Part model, mm, in its own coordinate system. Round coordinates to 2 decimals unless told otherwise and drop trailing zeros. Write each loop counter-clockwise with the first axis right and the second up, starting at its lowest first coordinate (ties: lowest second). Pieces come first, ordered by that corner, then holes. Notation, with made-up numbers: (-36.75, 35) -> (-30.75, 35) arc R16 cw to (-30.75, 50) -> close; hole circle Ø11 at (43.25, 78). An arc over 180 degrees is marked (long way). Return JSON: item names as keys, results as strings. Group by question number.
(1) Drop flat-ended pins along their axis: pin 1 Ø1 at (y, z) = (4, 23.5) entering from +X; pin 2 Ø2 at (y, z) = (2.5, -29) entering from -X; pin 3 Ø3 at (x, y) = (33.5, 4.5) entering from +Z; pin 4 Ø10 at (x, z) = (0, 31.75) entering from -Y. Give the stop position or say it passes through.
(2) Drill centre lines: L1, parallel to Z at x = 0.5, y = 4; L2, parallel to X at y = 2, z = 18.5; L3, parallel to Z at x = 4.5, y = 2.5. Where is each one in solid material? Low to high. Write a range as from..to.
(3) Saw through at A-A (z = 6.35). List the corners of the cut face in (x, y) (3 decimals).
from build123d import *

# Parameters (mm, degrees)
SKETCH1_R           = 3.175
SKETCH1_R_2         = 8.73125
BOSS_EXTRUDE1_DEPTH = 6.35
FILLET2_R           = 12.7
FILLET3_R           = 2.116666667
SKETCH2_R           = 10.2489
CUT_EXTRUDE1_DEPTH  = 1.27


with BuildPart() as part:
    # Sketch1 → Boss-Extrude1 (new body)
    with BuildSketch(Plane(origin=(0, 0, 0), x_dir=(1, 0, 0), z_dir=(0, 1, 0))):
        with BuildLine():
            Line((-12.7, 17.550968343), (-12.7, -44.45))
            Line((-12.7, -44.45), (12.7, -44.45))
            Line((12.7, -44.45), (12.7, 17.550968343))
            ThreePointArc((12.7, 17.550968343), (17.599905094, 24.459880613), (19.020487692, 32.80997545))
            Line((19.020487692, 32.80997545), (53.881536726, 67.671024484))
            Line((53.881536726, 67.671024484), (35.921024484, 85.631536726))
            Line((35.921024484, 85.631536726), (1.05997545, 50.770487692))
            ThreePointArc((1.05997545, 50.770487692), (-17.599905094, 39.040119387), (-12.7, 17.550968343))
        make_face()
        with Locations(Location((0, -31.75, 0), (0, 0, 270))):
            Circle(SKETCH1_R, mode=Mode.SUBTRACT)
        with Locations(Location((0, -6.35, 0), (0, 0, 270))):
            Circle(SKETCH1_R, mode=Mode.SUBTRACT)
        with Locations(Location((0, 31.75, 0), (0, 0, 270))):
            Circle(SKETCH1_R_2, mode=Mode.SUBTRACT)
        with Locations(Location((35.921024484, 67.671024484, 0), (0, 0, 270))):
            Circle(SKETCH1_R, mode=Mode.SUBTRACT)
        with Locations(Location((15.875, 47.625, 0), (0, 0, 270))):
            Circle(SKETCH1_R, mode=Mode.SUBTRACT)
    extrude(amount=BOSS_EXTRUDE1_DEPTH)

    # Fillet2
    fillet2_edges = [part.edges().sort_by_distance(p)[0] for p in [
        (35.921024484, 3.175, -85.631536726),
        (53.881536726, 3.175, -67.671024484),
        (-12.7, 3.175, 44.45),
        (12.7, 3.175, 44.45),
        (1.05997545, 3.175, -50.770487692),
        (-12.7, 3.175, -17.550968343),
        (12.7, 3.175, -17.550968343),
        (19.020487692, 3.175, -32.80997545),
    ]]
    fillet(fillet2_edges, radius=FILLET2_R - 0.0001)  # a hair under: the kernel refuses the full size

    # Fillet3
    fillet3_edges = [part.edges().sort_by_distance(p)[0] for p in [
        (17.599905094, 0, -24.459880613),
        (17.599905094, 6.35, -24.459880613),
        (12.7, 0, 9.525033333),
        (12.7, 6.35, 9.525033333),
        (33.675984024, 0, -47.465471782),
        (33.675984024, 6.35, -47.465471782),
        (-17.599905094, 0, -39.040119387),
        (-17.599905094, 6.35, -39.040119387),
        (15.715471782, 0, -65.425984024),
        (15.715471782, 6.35, -65.425984024),
        (-12.7, 0, 9.525033333),
        (-12.7, 6.35, 9.525033333),
        (8.98028541, 0, 40.73028541),
        (-8.98028541, 0, 40.73028541),
        (48.621065906, 0, -67.671024484),
        (35.921024484, 0, -80.371065906),
        (8.98028541, 6.35, 40.73028541),
        (-8.98028541, 6.35, 40.73028541),
        (48.621065906, 6.35, -67.671024484),
        (35.921024484, 6.35, -80.371065906),
        (13.351719091, 0, -16.716100664),
        (13.351719091, 6.35, -16.716100664),
        (20.071663278, 0, -32.939481059),
        (20.071663278, 6.35, -32.939481059),
        (1.189481059, 0, -51.821663278),
        (1.189481059, 6.35, -51.821663278),
        (-13.351719091, 0, -16.716100664),
        (-13.351719091, 6.35, -16.716100664),
    ]]
    fillet(fillet3_edges, radius=FILLET3_R)

    # Sketch2 → Cut-Extrude1 (cut)
    with BuildSketch(Plane(origin=(0, 6.35, 0), x_dir=(1, 0, 0), z_dir=(0, 1, 0))):
        with Locations(Location((0, 31.75, 0), (0, 0, 270))):
            Circle(SKETCH2_R)
    extrude(amount=-CUT_EXTRUDE1_DEPTH, mode=Mode.SUBTRACT)


solid = part.part
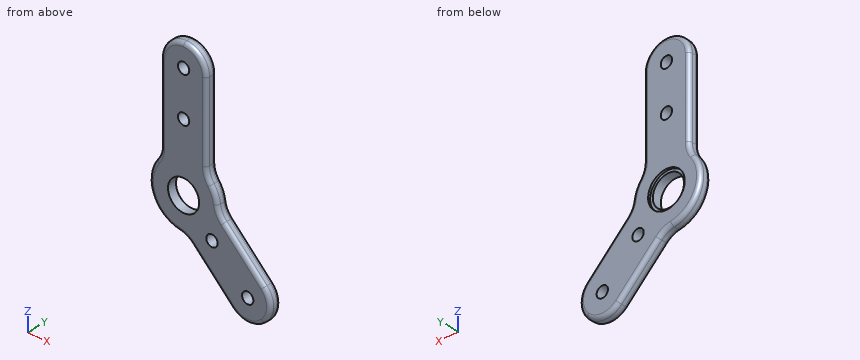
Computed values:
{
 "1": {"pin 1": "x = 12.7", "pin 2": "x = -18.97", "pin 3": "z = -45.8", "pin 4": "y = 0"},
 "2": {"L1": "-51.5..-40.47, -23.03..3.21, 9.49..28.61, 34.89..44.44", "L2": "-12.7..12.7", "L3": "-54.21..-39.23, -24.27..43.63"},
 "3": {"outline": "(-12.7, 2.117) arc R2.117 ccw to (-10.583, 0) -> (-3.175, 0) -> (-3.175, 6.35) -> (-10.583, 6.35) arc R2.117 ccw to (-12.7, 4.233) -> close; (3.175, 0) -> (10.583, 0) arc R2.117 ccw to (12.7, 2.117) -> (12.7, 4.233) arc R2.117 ccw to (10.583, 6.35) -> (3.175, 6.35) -> close"}
}
